Geometry: final body of the model. Coordinates: model frame, mm. Face numbers are marked on the shaded views. A direction names the side the tool comes from. Give positions to 0.01 mm unless a question says otherwise; leave off trailing zeros. Write each loop counter-clockwise with the first axis right and the second up, starting at its lowest first coordinate (ties: lowest second). Pieces come first, ordered by that corner, then holes. Notation, with made-up numbers: (19, 18.5) - (59, 18.5) arc R22 ccw to (59, 56.5) - close; hole circle Ø5 at (30.25, -4.75). An arc over 180 degrees is marked (long way). One line per question, with ' | ' between items. Start each with the question number.
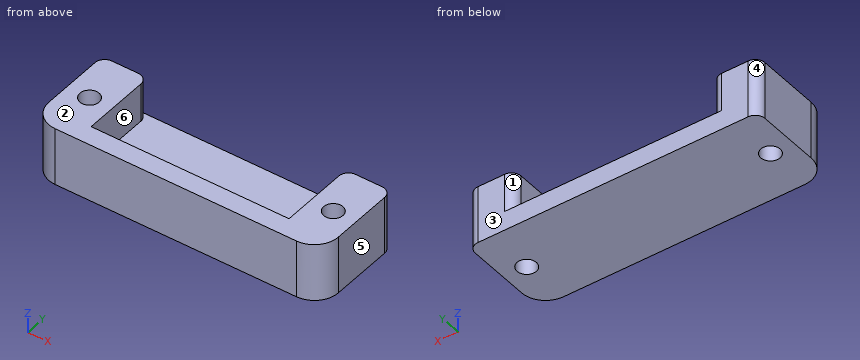
Autodesk Inventor part; units mm, degrees
ref_plane "YZ Plane" through (0, 0, 0) normal (1, 0, 0) x (0, 1, 0)
ref_plane "XZ Plane" through (0, 0, 0) normal (0, 1, 0) x (-1, 0, 0)
ref_plane "XY Plane" through (0, 0, 0) normal (0, 0, 1) x (1, 0, 0)
sketch "Sketch1" plane through (0, 0, 0) normal (0, 0, 1) x (1, 0, 0)
  line L0 (-30, 10) -> (30, 10)
  line L1 (30, 10) -> (30, -10)
  line L2 (30, -10) -> (-30, -10)
  line L3 (-30, -10) -> (-30, 10)
  line L4 (-30, 10) -> (30, -10) construction
  line L5 (30, 10) -> (-30, -10) construction
  point P0 (0, 0)
  dimension "d0" = 60
  dimension "d1" = 20
extrude "Extrusion1" add sketch "Sketch1" along normal blind 12
sketch "Sketch2" plane through (0, 0, 12) normal (0, 0, 1) x (1, 0, 0)
  line L0 (-20.5, -6) -> (20.5, -6)
  line L1 (20.5, -6) -> (20.5, 10)
  line L2 (20.5, 10) -> (-20.5, 10)
  line L3 (-20.5, 10) -> (-20.5, -6)
  line L4 (30, 10) -> (-30, 10)
  line L5 (-30, -10) -> (30, -10)
  point P0 (0, 0)
  point P1 (0, 10)
  dimension "d4" = 41
  dimension "d5" = 4
extrude "Extrusion2" cut sketch "Sketch2" against normal blind 8
sketch "Sketch3" plane through (0, 0, 12) normal (0, 0, 1) x (1, 0, 0)
  line L0 (-25.25, 0) -> (25.25, 0) construction
  line L1 (-30, 10) -> (-30, -10)
  line L2 (-20.5, -6) -> (-20.5, 10)
  point P0 (0, 0)
  point P1 (0, 0)
  dimension "d8" = 9.5
  dimension "d9" = 4.75
hole "Hole1" at (-25.25, 0, 12) at (25.25, 0, 12) direction (0, 0, -1) diameter 4 end through all
fillet "Fillet1" radius 2 4 edges at (-30, 10, 6) (-20.5, 10, 8) (20.5, 10, 8) (30, 10, 6)
fillet "Fillet2" radius 5 2 edges at (30, -10, 6) (-30, -10, 6)
equation "\"d9\" = 0.5 * d8"
properties part number "Battery Support"
1) Section D-D, the plane y = 7.25. Output: boundary loops of the cut face in (x, z).
2) Line query: L1, parallel to X at y = 0, z = 8.75; L2, parallel to X at y = 0, z = 2.5; L3, parallel to X at y = 7.25, z = 6.75. Output: solid intervals per line, ascending.
3) Reachability of the marked faces 1 and 2 from +Z, -Z, +X, -X, +Y, -Y: full face, straight path, thin tool, end or side. Return the list, or none.
4) Section C-C, the plane x = 4.5. Output: boundary loops of the cut face in (y, z).
5) Section A-A, the plane z = 6.5. Output: boundary loops of the cut face in (x, y).
6) Pull-direction query (X, two-part tool) for the marked faces 3, 4, 5 and 6; classes: +X half, -X half, draft (parallel to the pull), parting line (faces both ways), or undercut.
7) First-contact query: pin 1 Ø3 at (x, z) = (2, 10) entering from +Y; pin 2 Ø12 at (x, y) = (-12, 7) entering from +Z. Flat tips, straight axial feed; report the tip coordinate or a pass-through.
8) Section B-B, the plane y = 0. Output: boundary loops of the cut face in (x, z), plus the area to 3 significant figures.
Answer key:
1) outline: (-30, 0) - (30, 0) - (30, 12) - (20.5, 12) - (20.5, 4) - (-20.5, 4) - (-20.5, 12) - (-30, 12) - close
2) L1: -30 to -27.25, -23.25 to -20.5, 20.5 to 23.25, 27.25 to 30 | L2: -30 to -27.25, -23.25 to 23.25, 27.25 to 30 | L3: -30 to -20.5, 20.5 to 30
3) face 1: +Z, +Y | face 2: +Z, +X, -X, +Y, -Y
4) outline: (-10, 0) - (10, 0) - (10, 4) - (-6, 4) - (-6, 12) - (-10, 12) - close
5) outline: (-30, -5) arc R5 ccw to (-25, -10) - (25, -10) arc R5 ccw to (30, -5) - (30, 8) arc R2 ccw to (28, 10) - (22.5, 10) arc R2 ccw to (20.5, 8) - (20.5, -6) - (-20.5, -6) - (-20.5, 8) arc R2 ccw to (-22.5, 10) - (-28, 10) arc R2 ccw to (-30, 8) - close; hole circle Ø4 at (-25.25, 0); hole circle Ø4 at (25.25, 0)
6) face 3: draft | face 4: -X half | face 5: +X half | face 6: undercut
7) pin 1: y = -6 | pin 2: z = 4
8) outline: (-30, 0) - (-27.25, 0) - (-27.25, 12) - (-30, 12) - close; (-23.25, 0) - (23.25, 0) - (23.25, 12) - (20.5, 12) - (20.5, 4) - (-20.5, 4) - (-20.5, 12) - (-23.25, 12) - close; (27.25, 0) - (30, 0) - (30, 12) - (27.25, 12) - close | area: 296 mm^2
